from build123d import *

# Parameters (mm, degrees)
F0_R          = 63.246
F0_R_2        = 50.546
F1_DEPTH      = 19.05
F3_DEPTH      = 19.05
F4_W          = 1.5875
F4_H          = 19.0562327178
F5_DEPTH      = 19.051
F6_R          = 2.5527
F7_DEPTH      = 11.90625
F8_R          = 5.1417133043
F9_DEPTH      = 3.175
F9_DEPTH_BACK = 50.547
F11_D         = 3.7973
F12_W         = 22.225
F12_H         = 25.4
F13_DEPTH     = 19.05
F14_W         = 3.429
F14_H         = 15.621
F15_DEPTH     = 19.0510001
F16_T1_DEPTH  = 19.05
F16_T6_DEPTH  = 14.4190086939
F16_S7_R      = 5.1417133043
F16_T8_DEPTH  = 9
F16_T12_DEPTH = 14.4190086939
F16_S13_R     = 5.1417133043
F16_T14_DEPTH = 9
F16_T18_DEPTH = 17.6620719982
F16_S19_R     = 1.89865
F16_T20_DEPTH = 11
F16_T24_DEPTH = 17.6620719982
F16_S25_R     = 1.89865
F16_T26_DEPTH = 11
F16_T27_DEPTH = 44.45


# Not quite as in the source:
# - a fillet or chamfer that OpenCascade refuses, or shapes differently, is made with other operations: its cross-section is extruded or revolved along the edge and cut away or added


with BuildPart() as f1:
    # F0 (on Top) → F1 (new body)
    with BuildSketch(Plane.XY):
        Circle(F0_R)
        Circle(F0_R_2, mode=Mode.SUBTRACT)
    extrude(amount=F1_DEPTH)

    # F2 (on face) → F3 (join)
    with BuildSketch(Plane.XY.offset(19.05)):
        with BuildLine():
            Line((12.7, 69.596), (-12.7, 69.596))
            Line((-12.7, 69.596), (-12.7, 61.9577801087))
            ThreePointArc((-12.7, 61.9577801087), (0, 63.246), (12.7, 61.9577801087))
            Line((12.7, 61.9577801087), (12.7, 69.596))
        make_face()
    extrude(amount=-F3_DEPTH)

    # F4 (on face) → F5 (cut, through all)
    with BuildSketch(Plane.XY.offset(19.05)):
        with Locations((0, 60.0678836411)):
            Rectangle(F4_W, F4_H)
    extrude(amount=-F5_DEPTH, mode=Mode.SUBTRACT)

    # F6 (on face) → F7 (cut, through all)
    with BuildSketch(Plane.YZ.offset(12.7)):
        with Locations((61.9577801087, 9.525)):
            Circle(F6_R)
    extrude(amount=-F7_DEPTH, mode=Mode.SUBTRACT)

    # F8 (on face) → F9 (cut, two sides)
    with BuildSketch(Plane.YZ.offset(12.7)) as f9_sk:
        with Locations((61.9577801087, 9.525)):
            Circle(F8_R)
    extrude(amount=-F9_DEPTH, mode=Mode.SUBTRACT)
    extrude(f9_sk.sketch, amount=F9_DEPTH_BACK, mode=Mode.SUBTRACT)

    # F11 (through all)
    with Locations(Plane.YZ.offset(-0.79375)):
        with Locations((61.9577801087, 9.525)):
            Hole(F11_D / 2)

    # F12 (on face) → F13 (join)
    with BuildSketch(Plane.XY.offset(19.05)):
        with Locations((61.6585, 0)):
            Rectangle(F12_W, F12_H)
    extrude(amount=-F13_DEPTH)

    # F14 (on face) → F15 (cut, through all)
    with BuildSketch(Plane.XY.offset(19.05)):
        with Locations((61.5315, 0)):
            Rectangle(F14_W, F14_H)
    extrude(amount=-F15_DEPTH, mode=Mode.SUBTRACT)

    # F16: fillet of radius 5.08 on 8 edges, made by hand

    # F16_s2 → F16_t1 (join)
    with BuildSketch(Plane.XY):
        with BuildLine():
            ThreePointArc((61.0670823721, -16.4580669145), (62.882491273, -13.7475181293), (65.972068908, -12.7))
            Line((65.972068908, -12.7), (61.9577801087, -12.7))
            ThreePointArc((61.9577801087, -12.7), (61.5411241678, -14.585833955), (61.0670823721, -16.4580669145))
        make_face()
        with BuildLine():
            ThreePointArc((65.972068908, 12.7), (62.882491273, 13.7475181293), (61.0670823721, 16.4580669145))
            ThreePointArc((61.0670823721, 16.4580669145), (61.5411241678, 14.585833955), (61.9577801087, 12.7))
            Line((61.9577801087, 12.7), (65.972068908, 12.7))
        make_face()
    extrude(amount=F16_T1_DEPTH)


with BuildPart() as f16_tool4:
    # F16_s5 → F16_t6 (new body)
    with BuildSketch(Plane.XY.offset(19.05)):
        with BuildLine():
            ThreePointArc((16.4580669145, 61.0670823721), (13.7475181293, 62.882491273), (12.7, 65.972068908))
            Line((12.7, 65.972068908), (12.7, 61.9577801087))
            ThreePointArc((12.7, 61.9577801087), (14.585833955, 61.5411241678), (16.4580669145, 61.0670823721))
        make_face()
    extrude(amount=-F16_T6_DEPTH)

    # F16_s7 → F16_t8 (cut, symmetric)
    with BuildSketch(Plane.YZ.offset(14.6)):
        with Locations((61.9577801087, 9.525)):
            Circle(F16_S7_R)
    extrude(amount=F16_T8_DEPTH, both=True, mode=Mode.SUBTRACT)


with BuildPart() as f1_1:
    add(f1.part)

    # F16_t3: union F16_tool4
    add(f16_tool4.part)


with BuildPart() as f16_tool10:
    # F16_s11 → F16_t12 (new body)
    with BuildSketch(Plane.XY.offset(14.4190086939)):
        with BuildLine():
            ThreePointArc((16.4580669145, 61.0670823721), (13.7475181293, 62.882491273), (12.7, 65.972068908))
            Line((12.7, 65.972068908), (12.7, 61.9577801087))
            ThreePointArc((12.7, 61.9577801087), (14.585833955, 61.5411241678), (16.4580669145, 61.0670823721))
        make_face()
    extrude(amount=-F16_T12_DEPTH)

    # F16_s13 → F16_t14 (cut, symmetric)
    with BuildSketch(Plane.YZ.offset(14.6)):
        with Locations((61.9577801087, 9.525)):
            Circle(F16_S13_R)
    extrude(amount=F16_T14_DEPTH, both=True, mode=Mode.SUBTRACT)


with BuildPart() as f1_2:
    add(f1_1.part)

    # F16_t9: union F16_tool10
    add(f16_tool10.part)


with BuildPart() as f16_tool16:
    # F16_s17 → F16_t18 (new body)
    with BuildSketch(Plane.XY.offset(19.05)):
        with BuildLine():
            ThreePointArc((-16.4580669145, 61.0670823721), (-13.7475181293, 62.882491273), (-12.7, 65.972068908))
            Line((-12.7, 65.972068908), (-12.7, 61.9577801087))
            ThreePointArc((-12.7, 61.9577801087), (-14.585833955, 61.5411241678), (-16.4580669145, 61.0670823721))
        make_face()
    extrude(amount=-F16_T18_DEPTH)

    # F16_s19 → F16_t20 (cut, symmetric)
    with BuildSketch(Plane.YZ.offset(-14.6)):
        with Locations((61.9577801087, 9.525)):
            Circle(F16_S19_R)
    extrude(amount=F16_T20_DEPTH, both=True, mode=Mode.SUBTRACT)


with BuildPart() as f1_3:
    add(f1_2.part)

    # F16_t15: union F16_tool16
    add(f16_tool16.part)


with BuildPart() as f16_tool22:
    # F16_s23 → F16_t24 (new body)
    with BuildSketch(Plane.XY.offset(17.6620719982)):
        with BuildLine():
            ThreePointArc((-16.4580669145, 61.0670823721), (-13.7475181293, 62.882491273), (-12.7, 65.972068908))
            Line((-12.7, 65.972068908), (-12.7, 61.9577801087))
            ThreePointArc((-12.7, 61.9577801087), (-14.585833955, 61.5411241678), (-16.4580669145, 61.0670823721))
        make_face()
    extrude(amount=-F16_T24_DEPTH)

    # F16_s25 → F16_t26 (cut, symmetric)
    with BuildSketch(Plane.YZ.offset(-14.6)):
        with Locations((61.9577801087, 9.525)):
            Circle(F16_S25_R)
    extrude(amount=F16_T26_DEPTH, both=True, mode=Mode.SUBTRACT)


with BuildPart() as f1_4:
    add(f1_3.part)

    # F16_t21: union F16_tool22
    add(f16_tool22.part)

    # F16_s28 → F16_t27 (cut)
    with BuildSketch(Plane.XY.offset(-12.7)):
        with BuildLine():
            ThreePointArc((67.691, -12.7), (71.2831024484, -11.2121024484), (72.771, -7.62))
            Line((72.771, -7.62), (72.771, -12.7))
            Line((72.771, -12.7), (67.691, -12.7))
        make_face()
        with BuildLine():
            ThreePointArc((72.771, 7.62), (71.2831024484, 11.2121024484), (67.691, 12.7))
            Line((67.691, 12.7), (72.771, 12.7))
            Line((72.771, 12.7), (72.771, 7.62))
        make_face()
    extrude(amount=F16_T27_DEPTH, mode=Mode.SUBTRACT)


solid = f1_4.part
The listing builds one solid part. Answer for the finished solid, in the listing's coordinates (mm). A direction names the side the tool comes from. Give positions to 0.01 mm unless a question says otherwise; leave off trailing zeros. Loops run counter-clockwise (first coordinate to the right, second up) from the corner with the lowest first, then second, coordinate; pieces in that order, holes last. Notation, with made-up numbers: (62, 8) - (77, 8) arc R12 cw to (77, 27) - close; hole circle Ø1 at (1.5, 41). An arc over 180 degrees is marked (long way). Answer as a JSON object with one key per item and string values.
1. For a pull along Y with two mould halves and no side action, classify faces 4 (the cylindrical face through (5.22, 59.408, 9.637)), 5 (the flat face through (50.4, -6.4, 19.05)), 6 (the cylindrical face through (45.05, 44.39, 9.39)) as pulls with the +Y half, pulls with the -Y half, needs draft (parallel to the pull), parting line crosses it, or undercut.
Determined:
{"face 4": "undercut", "face 5": "needs draft", "face 6": "pulls with the +Y half"}
2. A cutting plane is placed at A-A (z = 16.25). Write down the section's boundary in (x, y).
Determined:
{"outline": "(-16.46, 61.07) arc R63.25 ccw (long way) to (61.07, -16.46) arc R5.08 cw to (65.97, -12.7) - (67.69, -12.7) arc R5.08 ccw to (72.77, -7.62) - (72.77, 7.62) arc R5.08 ccw to (67.69, 12.7) - (65.97, 12.7) arc R5.08 cw to (61.07, 16.46) arc R63.25 ccw to (16.46, 61.07) arc R5.08 cw to (12.7, 65.97) - (12.7, 69.6) - (0.79, 69.6) - (0.79, 50.54) arc R50.55 cw (long way) to (-0.79, 50.54) - (-0.79, 69.6) - (-12.7, 69.6) - (-12.7, 65.97) arc R5.08 cw to start; hole (59.82, -7.81) - (63.25, -7.81) - (63.25, 7.81) - (59.82, 7.81) - close"}
3. A cutting plane is placed at C-C (x = -52.5). Write down the section's boundary in (y, z), then the cut area to 3 significant figures.
Determined:
{"outline": "(-35.27, 0) - (35.27, 0) - (35.27, 19.05) - (-35.27, 19.05) - close", "area": "1,340 mm²"}
4. A cutting plane is placed at B-B (y = -37). Write down the section's boundary in (x, z), then the cut area to 3 significant figures.
Determined:
{"outline": "(-51.29, 0) - (-34.44, 0) - (-34.44, 19.05) - (-51.29, 19.05) - close; (34.44, 0) - (51.29, 0) - (51.29, 19.05) - (34.44, 19.05) - close", "area": "642 mm²"}
5. Find the intervals of material crossed by L1, parallel to X at y = 0, z = 10.75; L2, parallel to X at y = 35.5, z = 16.5; L3, parallel to Y at x = 10, z = 14.75, in increasing order. Write a range as [from, to].
Determined:
{"L1": "[-63.25, -50.55], [50.55, 59.82], [63.25, 72.77]", "L2": "[-52.34, -35.98], [35.98, 52.34]", "L3": "[-62.45, -49.55], [49.55, 69.6]"}
6. Flat-ended cylindrical pins translate along their axes: pin 1 Ø3 at (y, z) = (68, 12.5) entering from -X; pin 2 Ø3 at (y, z) = (67, 5.5) entering from +X; pin 3 Ø10 at (y, z) = (-12, 9) entering from -X; pin 4 Ø5 at (x, y) = (56.5, 22.5) entering from -Z. Find the tip coordinate at first contact, or state that the pin passes through.
Determined:
{"pin 1": "x = -12.7", "pin 2": "x = 12.72", "pin 3": "x = -62.86", "pin 4": "z = 0"}
7. For faces 1 (the flat face through (12.7, 68, 10)), 2 (the flat face through (-12.7, 68, 10)), 3 (the flat face through (63.246, 0, 10)), determine the directions among +Z, -Z, +X, -X, +Y, -Y from which every point of the face is accessible in a straight line to the end or side of a thin tool.
Determined:
{"face 1": "+Z, -Z, +X, +Y", "face 2": "+Z, -Z, -X, +Y", "face 3": "+Z, -Z"}
